from build123d import *

# Parameters (mm, degrees)
F0_W     = 142
F0_H     = 142
F1_DEPTH = 5.2
F0_W_2   = 124.5
F0_H_2   = 123.5
F2_DEPTH = 20.4


with BuildPart() as f1:
    # F0 (on Top) → F1 (new body)
    with BuildSketch(Plane.XY):
        Rectangle(F0_W, F0_H)
        with BuildLine():
            Line((-63.75, 66.25), (63.75, 66.25))
            ThreePointArc((63.75, 66.25), (65.87132, 65.37132), (66.75, 63.25))
            Line((66.75, 63.25), (66.75, -63.25))
            ThreePointArc((66.75, -63.25), (65.87132, -65.37132), (63.75, -66.25))
            Line((63.75, -66.25), (-63.75, -66.25))
            ThreePointArc((-63.75, -66.25), (-65.87132, -65.37132), (-66.75, -63.25))
            Line((-66.75, -63.25), (-66.75, 63.25))
            ThreePointArc((-66.75, 63.25), (-65.87132, 65.37132), (-63.75, 66.25))
        make_face(mode=Mode.SUBTRACT)
    extrude(amount=-F1_DEPTH)

    # F0 (on Top) → F2 (join)
    with BuildSketch(Plane.XY):
        with BuildLine():
            ThreePointArc((66.75, 63.25), (65.87132, 65.37132), (63.75, 66.25))
            Line((63.75, 66.25), (-63.75, 66.25))
            ThreePointArc((-63.75, 66.25), (-65.87132, 65.37132), (-66.75, 63.25))
            Line((-66.75, 63.25), (-66.75, -63.25))
            ThreePointArc((-66.75, -63.25), (-65.87132, -65.37132), (-63.75, -66.25))
            Line((-63.75, -66.25), (63.75, -66.25))
            ThreePointArc((63.75, -66.25), (65.87132, -65.37132), (66.75, -63.25))
            Line((66.75, -63.25), (66.75, 63.25))
        make_face()
        Rectangle(F0_W_2, F0_H_2, mode=Mode.SUBTRACT)
    extrude(amount=-F2_DEPTH)


solid = f1.part
Work out the finished part from the listing and answer in its coordinate system (mm). A direction names the side the tool comes from. Coordinates: 2 decimals unless noted, no trailing zeros. Write each loop counter-clockwise with the first axis right and the second up, starting at its lowest first coordinate (ties: lowest second). Pieces come first, ordered by that corner, then holes.
1. For faces 1 (the flat face through (-1, 61.75, -10)), 2 (the flat face through (-6, -68, -5.2)), 3 (the flat face through (1, 66.25, -13)), determine the directions among +Z, -Z, +X, -X, +Y, -Y from which every point of the face is accessible in a straight line to the end or side of a thin tool.
Results list:
face 1: +Z, -Z
face 2: -Z
face 3: -Z, +X, -X, +Y
2. The part is cut by section D-D, the plane z = -16.5. Write down the section's boundary in (x, y).
Results list:
outline: (-66.75, -63.25) arc R3 ccw to (-63.75, -66.25) - (63.75, -66.25) arc R3 ccw to (66.75, -63.25) - (66.75, 63.25) arc R3 ccw to (63.75, 66.25) - (-63.75, 66.25) arc R3 ccw to (-66.75, 63.25) - close; hole (-62.25, -61.75) - (62.25, -61.75) - (62.25, 61.75) - (-62.25, 61.75) - close
3. The part is cut by section A-A, the plane x = -3. Write down the section's boundary in (y, z).
Results list:
outline: (-71, -5.2) - (-66.25, -5.2) - (-66.25, -20.4) - (-61.75, -20.4) - (-61.75, 0) - (-71, 0) - close; (61.75, -20.4) - (66.25, -20.4) - (66.25, -5.2) - (71, -5.2) - (71, 0) - (61.75, 0) - close
4. Flat-ended cylindrical pins translate along their axes: pin 1 (10 mm diameter, centred on y = -3.5, z = -10.5, fed in from +X); pin 2 (6 mm diameter, centred on x = -7.5, z = -8.5, fed in from -Y); pin 3 (12 mm diameter, centred on y = 30, z = -12, fed in from -X). Find the tip coordinate at first contact, or state that the pin passes through.
Results list:
pin 1: stops at x = 66.75
pin 2: stops at y = -66.25
pin 3: stops at x = -66.75
5. Consider line 1 along Y through (x, z) = (-46, -9.5); line 2 along X through (y, z) = (9.5, -1.5); line 3 along X through (y, z) = (57, -6). Determine where each line is inside the solid, lowest interval first.
Results list:
line 1: y = -66.25 to -61.75, 61.75 to 66.25
line 2: x = -71 to -62.25, 62.25 to 71
line 3: x = -66.75 to -62.25, 62.25 to 66.75
6. For a pull along X with two mould halves and no side action, classify faces 4 (the flat face through (-66.75, 1, -13)), 5 (the flat face through (-62.25, -1, -10)), 6 (the flat face through (66.75, -1, -13)) as +X half, -X half, draft (parallel to the pull), parting line (faces both ways), or undercut.
Results list:
face 4: -X half
face 5: undercut
face 6: +X half
7. The part is cut by section B-B, the plane y = 46. Write down the section's boundary in (x, z), and give its area (3 significant figures).
Results list:
outline: (-71, -5.2) - (-66.75, -5.2) - (-66.75, -20.4) - (-62.25, -20.4) - (-62.25, 0) - (-71, 0) - close; (62.25, -20.4) - (66.75, -20.4) - (66.75, -5.2) - (71, -5.2) - (71, 0) - (62.25, 0) - close
area: 228 mm2
8. The part is cut by section C-C, the plane z = -2.5. Write down the section's boundary in (x, y).
Results list:
outline: (-71, -71) - (71, -71) - (71, 71) - (-71, 71) - close; hole (-62.25, -61.75) - (62.25, -61.75) - (62.25, 61.75) - (-62.25, 61.75) - close
